```python
from build123d import *

# Parameters (mm, degrees)
SKETCH2_R                       = 65.405
BOSS_EXTRUDE1_DEPTH             = 6.35
SKETCH4_R                       = 65.405
SKETCH4_R_2                     = 61.595
CUT_EXTRUDE1_DEPTH              = 3.175
F_1_4_0_25_DIAMETER_HOLE1_D     = 6.35
F_13_16_0_8125_DIAMETER_HOLE1_D = 20.6375
CUT_EXTRUDE3_DEPTH              = 3.175
SKETCH9_R                       = 6.0325
CUT_EXTRUDE2_DEPTH              = 1.5875


with BuildPart() as part:
    # Sketch2 → Boss-Extrude1 (new body)
    with BuildSketch(Plane(origin=(0, 0, 0), x_dir=(1, 0, 0), z_dir=(0, 1, 0))):
        Circle(SKETCH2_R)
    extrude(amount=BOSS_EXTRUDE1_DEPTH)

    # Sketch4 → Cut-Extrude1 (cut)
    with BuildSketch(Plane(origin=(0, 6.35, 0), x_dir=(1, 0, 0), z_dir=(0, 1, 0))):
        Circle(SKETCH4_R)
        Circle(SKETCH4_R_2, mode=Mode.SUBTRACT)
    extrude(amount=-CUT_EXTRUDE1_DEPTH, mode=Mode.SUBTRACT)

    # 1/4 (0.25) Diameter Hole1 (through all)
    with Locations(Plane(origin=(0, 6.35, 0), x_dir=(1, 0, 0), z_dir=(0, 1, 0))):
        with Locations((-33.675960454, 33.675960454), (-33.675960454, -33.675960454), (33.675960454, 33.675960454), (33.675960454, -33.675960454)):
            Hole(F_1_4_0_25_DIAMETER_HOLE1_D / 2)

    # 13/16 (0.8125) Diameter Hole1 (through all)
    with Locations(Plane(origin=(0, 6.35, 0), x_dir=(1, 0, 0), z_dir=(0, 1, 0))):
        with Locations((0, 0)):
            Hole(F_13_16_0_8125_DIAMETER_HOLE1_D / 2)

    # Sketch11 → Cut-Extrude3 (cut)
    with BuildSketch(Plane(origin=(0, 6.35, 0), x_dir=(1, 0, 0), z_dir=(0, 1, 0))):
        with BuildLine():
            Line((-5.601020514, 10.2), (5.601020514, 10.2))
            ThreePointArc((5.601020514, 10.2), (7.490842879, 10.570899501), (9.100291576, 11.628571429))
            ThreePointArc((9.100291576, 11.628571429), (11.914213562, 11.614213562), (11.928571429, 8.800291576))
            ThreePointArc((11.928571429, 8.800291576), (10.870899501, 7.190842879), (10.5, 5.301020514))
            Line((10.5, 5.301020514), (10.5, -25.901020514))
            ThreePointArc((10.5, -25.901020514), (10.870899501, -27.790842879), (11.928571429, -29.400291576))
            ThreePointArc((11.928571429, -29.400291576), (11.914213562, -32.214213562), (9.100291576, -32.228571429))
            ThreePointArc((9.100291576, -32.228571429), (7.490842879, -31.170899501), (5.601020514, -30.8))
            Line((5.601020514, -30.8), (-5.601020514, -30.8))
            ThreePointArc((-5.601020514, -30.8), (-7.490842879, -31.170899501), (-9.100291576, -32.228571429))
            ThreePointArc((-9.100291576, -32.228571429), (-11.914213562, -32.214213562), (-11.928571429, -29.400291576))
            ThreePointArc((-11.928571429, -29.400291576), (-10.870899501, -27.790842879), (-10.5, -25.901020514))
            Line((-10.5, -25.901020514), (-10.5, 5.301020514))
            ThreePointArc((-10.5, 5.301020514), (-10.870899501, 7.190842879), (-11.928571429, 8.800291576))
            ThreePointArc((-11.928571429, 8.800291576), (-11.914213562, 11.614213562), (-9.100291576, 11.628571429))
            ThreePointArc((-9.100291576, 11.628571429), (-7.490842879, 10.570899501), (-5.601020514, 10.2))
        make_face()
    extrude(amount=-CUT_EXTRUDE3_DEPTH, mode=Mode.SUBTRACT)

    # Sketch9 → Cut-Extrude2 (cut)
    with BuildSketch(Plane.XZ):
        with Locations((-33.675960454, 33.675960454)):
            Circle(SKETCH9_R)
        with Locations((33.675960454, 33.675960454)):
            Circle(SKETCH9_R)
        with Locations((33.675960454, -33.675960454)):
            Circle(SKETCH9_R)
        with Locations((-33.675960454, -33.675960454)):
            Circle(SKETCH9_R)
    extrude(amount=-CUT_EXTRUDE2_DEPTH, mode=Mode.SUBTRACT)


solid = part.part
```
Could you check a few things on this model? Use its own coordinates, in mm. A direction names the side the tool comes from. Give positions to 0.01 mm unless a question says otherwise; leave off trailing zeros. Order: outer loops, then holes, each group sorted by start corner. A loop starts at its lowest first (then second) coordinate and runs counter-clockwise, first axis right, second up.
Q1. If I drill on line 1 along Z through (x, y) = (33, 0.5); line 2 along X through (y, z) = (6, -31.5); line 3 along Z through (x, y) = (36, 2.75), over which ranges is the centre line in solid material (lowest first)?
Q2. We'd pull the mould along X, two halves only. Please class faces 1 (the flat face through (58, 3.175, 24)), 2 (the cylindrical face through (-10.881, 4.785, 27.816)), 3 (the cylindrical face through (-13.35, 4.78, 60.13)): +X half, -X half, draft (parallel to the pull), parting line (faces both ways), or undercut.
Q3. Suppose I cut it at B-B, the plane z = 5.5. Write out the boundary of the cut face in (x, y) (3 decimals), and give its area (3 significant figures).
Q4. Suppose I cut it at A-A, the plane x = 0. Write out the boundary of the cut face in (y, z) (3 decimals).
Q5. For faces 4 (the flat face through (-1, 0, 14)), 5 (the flat face through (-10.5, 5, 11)), 6 (the flat face through (-31, 1.588, -36)), which set-ups out of +Z, -Z, +X, -X, +Y, -Y let a thin tool reach every point of the face, with its end or its side?
Q6. I'm going to push flat-ended pins straight in: P1, Ø6, axis at x = -35.5, z = -35.5, coming from the -Y side; P2, Ø3, axis at y = 5.5, z = -46, coming from the -X side; P3, Ø7.5, axis at x = 3.5, z = 19.5, coming from the +Y side (3 decimals). Where does each tip first touch, or does it pass through?
Q7. Suppose I cut it at C-C, the plane y = 5.25. Count the separate pieces of the cut face and the enclosed holes in it, and give its area (3 significant figures).
Solution:
1. line 1: z = -56.47 to -39.67, -27.68 to 27.68, 39.67 to 56.47
1. line 2: x = -52.93 to -35.99, -31.36 to 31.36, 35.99 to 52.93
1. line 3: z = -54.61 to -35.84, -31.51 to 31.51, 35.84 to 54.61
2. face 1: draft
2. face 2: undercut
2. face 3: parting line
3. outline: (-65.173, 0) - (-8.731, 0) - (-8.731, 3.175) - (-10.5, 3.175) - (-10.5, 6.35) - (-61.349, 6.35) - (-61.349, 3.175) - (-65.173, 3.175) - close; (8.731, 0) - (65.173, 0) - (65.173, 3.175) - (61.349, 3.175) - (61.349, 6.35) - (10.5, 6.35) - (10.5, 3.175) - (8.731, 3.175) - close
3. area: 681 mm2
4. outline: (0, -65.405) - (3.175, -65.405) - (3.175, -61.595) - (6.35, -61.595) - (6.35, -10.319) - (0, -10.319) - close; (0, 10.319) - (3.175, 10.319) - (3.175, 30.8) - (6.35, 30.8) - (6.35, 61.595) - (3.175, 61.595) - (3.175, 65.405) - (0, 65.405) - close
5. face 4: +Z, -Z, +X, -X, -Y
5. face 5: +Y
5. face 6: -Y
6. P1: stops at y = 1.59
6. P2: stops at x = -42.59
6. P3: stops at y = 3.175
7. separate pieces: 1
7. enclosed holes: 5
7. area: 10,900 mm2
